```python
from build123d import *

# Parameters (mm, degrees)
PAD041_DEPTH    = 2
PAD042_DEPTH    = 2
POCKET014_DEPTH = 2.001


with BuildPart() as part:
    # Sketch064 → Pad041 (new body)
    with BuildSketch(Plane.XY):
        with BuildLine():
            Line((-5, 21), (5, 21))
            ThreePointArc((10, 16), (8.535534, 19.535534), (5, 21))
            Line((10, 16), (10, 1))
            Line((10, 1), (-10, 1))
            Line((-10, 1), (-10, 16))
            ThreePointArc((-5, 21), (-8.535534, 19.535534), (-10, 16))
        make_face()
        with BuildLine():
            ThreePointArc((-3, 16), (-5, 18), (-7, 16))
            Line((-7, 16), (-7, 11))
            ThreePointArc((-7, 11), (-5, 9), (-3, 11))
            Line((-3, 16), (-3, 11))
        make_face(mode=Mode.SUBTRACT)
        with BuildLine():
            ThreePointArc((7, 16), (5, 18), (3, 16))
            Line((3, 16), (3, 11))
            ThreePointArc((3, 11), (5, 9), (7, 11))
            Line((7, 16), (7, 11))
        make_face(mode=Mode.SUBTRACT)
    extrude(amount=PAD041_DEPTH)

    # Sketch065 → Pad042 (join)
    with BuildSketch(Plane.XY):
        with BuildLine():
            ThreePointArc((-3, 1.5), (-6, 4.5), (-9, 1.5))
            Line((-9, 1.5), (-9, -1.5))
            ThreePointArc((-9, -1.5), (-6, -4.5), (-3, -1.5))
            Line((-3, 1.5), (-3, -1.5))
        make_face()
        with BuildLine():
            ThreePointArc((9, 1.5), (6, 4.5), (3, 1.5))
            Line((3, 1.5), (3, -1.5))
            ThreePointArc((3, -1.5), (6, -4.5), (9, -1.5))
            Line((9, 1.5), (9, -1.5))
        make_face()
    extrude(amount=PAD042_DEPTH)

    # Sketch066 → Pocket014 (cut, through all)
    with BuildSketch(Plane.XY):
        with BuildLine():
            ThreePointArc((-4.2, 1.5), (-6, 3.3), (-7.8, 1.5))
            Line((-7.8, 1.5), (-7.8, -1.5))
            ThreePointArc((-7.8, -1.5), (-6, -3.3), (-4.2, -1.5))
            Line((-4.2, 1.5), (-4.2, -1.5))
        make_face()
        with BuildLine():
            ThreePointArc((7.8, 1.5), (6, 3.3), (4.2, 1.5))
            Line((4.2, 1.5), (4.2, -1.5))
            ThreePointArc((4.2, -1.5), (6, -3.3), (7.8, -1.5))
            Line((7.8, 1.5), (7.8, -1.5))
        make_face()
    extrude(amount=POCKET014_DEPTH, mode=Mode.SUBTRACT)


with BuildPart() as part_1:
    # Body013 placement: moved
    add(part.part.moved(Location((-16, 2, -8.5))))


solid = part_1.part
```
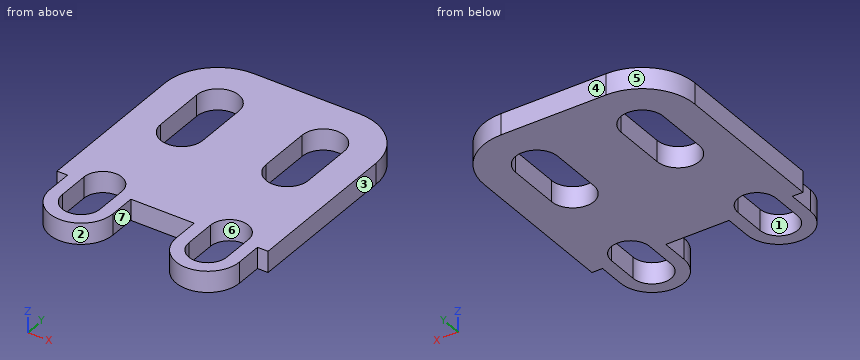
Verification items for the finished model (mm, model axes). Face numbers are marked on the shaded views. A direction names the side the tool comes from. Round coordinates to 2 decimals unless told otherwise and drop trailing zeros. Write each loop counter-clockwise with the first axis right and the second up, starting at its lowest first coordinate (ties: lowest second). Pieces come first, ordered by that corner, then holes. Notation, with made-up numbers: (34.5, 12.25) -> (61.5, 12.25) arc R17 cw to (61.5, 45.25) -> close; hole circle Ø3 at (57.25, 27). An arc over 180 degrees is marked (long way). Write each question's results on one line, items separated by ' | '. Start each with the question number.
1. Set-up check for the marked faces 5, 6 and 7: record each of +Z, -Z, +X, -X, +Y, -Y from which the full face is reachable in a straight line by a thin tool's end or side.
2. Depth check by flat-ended pin: P1, Ø0.6, axis at y = 2, z = -7.5, coming from the -X side; P2, Ø8, axis at x = -10.5, y = 0.5, coming from the -Z side; P3, Ø0.8, axis at x = -6.5, z = -8, coming from the -Y side. Enter the tip coordinate at first touch or a pass-through.
3. Cross-section at A-A (y = 17.25). Enter the section's corners in (x, z).
4. Draft check along X on the marked faces 1, 2, 3 and 4. Enter one of: +X half, -X half, draft (parallel to the pull), parting line (faces both ways), or undercut.
5. Material ranges on probe 1 along X at (y, z) = (16.75, -8.1); probe 2 along X at (y, z) = (2, -7.15); probe 3 along Y at (x, z) = (-11.5, -7.9), recorded low to high. Write a range as from..to.
6. Cross-section at D-D (x = -12.5). Enter the section's corners in (y, z), then the cut area to 3 significant figures.
7. Cross-section at C-C (y = -0.25). Enter the section's corners in (x, z), then the cut area to 3 significant figures.
8. Cross-section at B-B (z = -7.7). Count the separate pieces of the cut face and the enclosed holes in it, then the cut area to 3 significant figures.
Solutions:
1) face 5: +Z, -Z, -X, +Y | face 6: +Z, -Z | face 7: +Z, -Z, -Y
2) P1: stops at x = -25 | P2: stops at z = -8.5 | P3: stops at y = 3
3) outline: (-26, -8.5) -> (-23, -8.5) -> (-23, -6.5) -> (-26, -6.5) -> close; (-19, -8.5) -> (-13, -8.5) -> (-13, -6.5) -> (-19, -6.5) -> close; (-9, -8.5) -> (-6, -8.5) -> (-6, -6.5) -> (-9, -6.5) -> close
4) face 1: undercut | face 2: undercut | face 3: +X half | face 4: draft
5) probe 1: x = -26..-23, -19..-13, -9..-6 | probe 2: x = -25..-23.8, -20.2..-19, -13..-11.8, -8.2..-7 | probe 3: y = -2.1..-0.49, 4.49..11.06, 19.94..23
6) outline: (-1.16, -8.5) -> (11.68, -8.5) -> (11.68, -6.5) -> (-1.16, -6.5) -> close; (19.32, -8.5) -> (23, -8.5) -> (23, -6.5) -> (19.32, -6.5) -> close | area: 33.0 mm2
7) outline: (-24.9, -8.5) -> (-23.64, -8.5) -> (-23.64, -6.5) -> (-24.9, -6.5) -> close; (-20.36, -8.5) -> (-19.1, -8.5) -> (-19.1, -6.5) -> (-20.36, -6.5) -> close; (-12.9, -8.5) -> (-11.64, -8.5) -> (-11.64, -6.5) -> (-12.9, -6.5) -> close; (-8.36, -8.5) -> (-7.1, -8.5) -> (-7.1, -6.5) -> (-8.36, -6.5) -> close | area: 10.1 mm2
8) separate pieces: 1 | enclosed holes: 4 | area: 340 mm2
